For this review, take the finished solid that the model builds, in its own axes (mm). Round coordinates to 2 decimals unless told otherwise and drop trailing zeros. Loops run counter-clockwise (first coordinate to the right, second up) from the corner with the lowest first, then second, coordinate; pieces in that order, holes last.
1. To check wall thickness, follow line 1 along Y through (x, z) = (2, 636.5); line 2 along Y through (x, z) = (25, 375.5); line 3 along X through (y, z) = (15, 298.5). State the ranges of each line that lie inside material, in increasing order.
2. Clearance check with flat-ended pins moving along their axes: pin 1 Ø1 at (x, y) = (-1.5, 13) entering from -Z; pin 2 Ø10 at (x, z) = (-15, 344) entering from +Y; pin 3 Ø1.5 at (x, y) = (15.5, -22) entering from +Z. State where each tip first meets the part, or that it passes through.
3. Consider section B-B on x = 0. State the section outline as (y, z) points.
4. Consider section A-A on z = 591.5. State the section outline as (x, y) points.
5. Draft analysis for pull direction X (two halves, no side actions). For faces 1 (the cylindrical face through (-29.97, 1.32, 419.05)), 2 (the flat face through (0, 0, 30)), state which applies: released by +X, released by -X, zero draft, split by the parting line, or undercut.
6. Consider section C-C on y = 0. State the section outline as (x, z) points.
from build123d import *

# Parameters (mm, degrees)
SKETCH1_R           = 30
BOSS_EXTRUDE2_DEPTH = 850
CUT_EXTRUDE1_DEPTH  = 70
CUT_EXTRUDE2_DEPTH  = 70


with BuildPart() as part:
    # Sketch1 → Boss-Extrude2 (new body)
    with BuildSketch(Plane.XY):
        Circle(SKETCH1_R)
    extrude(amount=BOSS_EXTRUDE2_DEPTH)

    # Sketch4 → Cut-Extrude1 (cut)
    with BuildSketch(Plane(origin=(0, 40, 0), x_dir=(1, 0, 0), z_dir=(0, 1, 0))):
        Polygon((-30, -850), (30, -850), (30, -790), align=None)
    extrude(amount=-CUT_EXTRUDE1_DEPTH, mode=Mode.SUBTRACT)

    # Sketch3 → Cut-Extrude2 (cut)
    with BuildSketch(Plane(origin=(0, 40, 0), x_dir=(1, 0, 0), z_dir=(0, 1, 0))):
        Polygon((-30, 0), (30, -60), (30, 0), align=None)
    extrude(amount=-CUT_EXTRUDE2_DEPTH, mode=Mode.SUBTRACT)


solid = part.part
Resolved:
1. line 1: y = -29.93 to 29.93
1. line 2: y = -16.58 to 16.58
1. line 3: x = -25.98 to 25.98
2. pin 1: stops at z = 28
2. pin 2: stops at y = 28.28
2. pin 3: stops at z = 805.25
3. outline: (-30, 30) - (30, 30) - (30, 820) - (-30, 820) - close
4. outline: circle Ø60 at (0, 0)
5. face 1: split by the parting line
5. face 2: released by +X
6. outline: (-30, 0) - (30, 60) - (30, 790) - (-30, 850) - close
